Can you work these out from the model? Positions are in its coordinate system, mm. Face numbers are marked on the shaded views. A direction names the side the tool comes from. Give positions to 0.01 mm unless a question says otherwise; leave off trailing zeros. Order: outer loops, then holes, each group sorted by start corner. A loop starts at its lowest first (then second) coordinate and runs counter-clockwise, first axis right, second up.
Item 1: I want a section at C-C, the plane x = 16. Write out the boundary of the cut face in (y, z) (3 decimals), then the cut area to 3 significant figures.
Item 2: I want a section at D-D, the plane y = -21.5. Write out the boundary of the cut face in (x, z), then the cut area to 3 significant figures.
Item 3: I want a section at A-A, the plane x = 0. Write out the boundary of the cut face in (y, z) (3 decimals), then the cut area to 3 significant figures.
Item 4: I want a section at B-B, the plane z = 14. Write out the boundary of the cut face in (x, y) (3 decimals), then the cut area to 3 significant figures.
Item 5: If we mould it in two halves opening along X, with no side actions, what happens to the marked faces 1, 2 and 3? For each: +X half, -X half, draft (parallel to the pull), parting line (faces both ways), or undercut.
Item 6: I'm going to push flat-ended pins straight in: pin 1 Ø1.5 at (x, z) = (-40.5, 31) entering from +Y; pin 2 Ø12 at (x, y) = (17.5, 2) entering from -Z; pin 3 Ø15 at (x, z) = (-69.5, 25.5) entering from +Y; pin 4 Ø3 at (y, z) = (19.5, 28) entering from +X. Where does each tip first touch, or does it pass through?
Item 7: Which directions (+Z, -Z, +X, -X, +Y, -Y) give clear straight access to the entire face, cutting with the end or side of a thin tool? Please do the marked faces 4, 5 and 6.
Item 8: If I drill on line 1 along Y through (x, z) = (0, 8) (3 decimals); line 2 along Y through (x, z) = (-69, 12) (3 decimals); line 3 along X through (y, z) = (8.5, 17.5), over which ranges is the centre line in solid material (lowest first)?
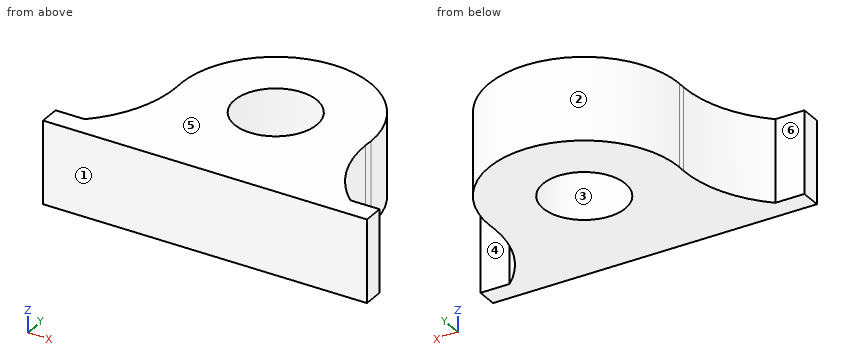
```python
from build123d import *

# Parameters (mm, degrees)
CROQUIS1_R              = 19
SALIENTE_EXTRUIR1_DEPTH = 38.1


with BuildPart() as part:
    # Croquis1 → Saliente-Extruir1 (new body)
    with BuildSketch(Plane.XY):
        with BuildLine():
            Line((-61.503424818, -44), (-75, -44))
            Line((-75, -44), (-75, -53.525))
            Line((-75, -53.525), (75, -53.525))
            Line((75, -53.525), (75, -44))
            Line((75, -44), (61.503424818, -44))
            ThreePointArc((61.503424818, -44), (48.377816196, -25.671153051), (43.853638254, -3.585862786))
            ThreePointArc((43.853638254, -3.585862786), (43.897102733, -1.791718479), (44, 0))
            ThreePointArc((44, 0), (0, 44), (-44, 0))
            ThreePointArc((-44, 0), (-43.897102733, -1.791718479), (-43.853638254, -3.585862786))
            ThreePointArc((-43.853638254, -3.585862786), (-48.377816196, -25.671153051), (-61.503424818, -44))
        make_face()
        with Locations(Location((0, 0, 0), (0, 0, 180))):
            Circle(CROQUIS1_R, mode=Mode.SUBTRACT)
    extrude(amount=SALIENTE_EXTRUIR1_DEPTH)


solid = part.part
```
Results list:
1. outline: (-53.525, 0) - (-10.247, 0) - (-10.247, 38.1) - (-53.525, 38.1) - close; (10.247, 0) - (40.988, 0) - (40.988, 38.1) - (10.247, 38.1) - close
1. area: 2,820 mm2
2. outline: (-46.76, 0) - (46.76, 0) - (46.76, 38.1) - (-46.76, 38.1) - close
2. area: 3,560 mm2
3. outline: (-53.525, 0) - (-19, 0) - (-19, 38.1) - (-53.525, 38.1) - close; (19, 0) - (44, 0) - (44, 38.1) - (19, 38.1) - close
3. area: 2,270 mm2
4. outline: (-75, -53.525) - (75, -53.525) - (75, -44) - (61.503, -44) arc R54.148 cw to (44, 0) arc R44 ccw to (-44, 0) arc R54.148 cw to (-61.503, -44) - (-75, -44) - close; hole circle Ø38 at (0, 0)
4. area: 7,630 mm2
5. face 1: draft
5. face 2: parting line
5. face 3: undercut
6. pin 1: stops at y = 18.87
6. pin 2: stops at z = 0
6. pin 3: stops at y = -44
6. pin 4: stops at x = 40.15
7. face 4: +Z, -Z, +X, +Y
7. face 5: +Z, +X, -X, +Y, -Y
7. face 6: +Z, -Z, -X, +Y
8. line 1: y = -53.525 to -19, 19 to 44
8. line 2: y = -53.525 to -44
8. line 3: x = -43.17 to -16.99, 16.99 to 43.17
